Part model, mm, in its own coordinate system. Coordinates: 2 decimals unless noted, no trailing zeros. Order: outer loops, then holes, each group sorted by start corner. A loop starts at its lowest first (then second) coordinate and runs counter-clockwise, first axis right, second up. Notation, with made-up numbers: M 48,11 L 60,11 A20 ccw 60,20 Z; hole C 40.5,64 d1. An arc over 180 degrees is marked long. Answer in a Markdown table with one row per item. Add a question column.
Autodesk Inventor part; units mm, degrees
ref_plane "Work Plane2" through (18, 0, 0) normal (1, 0, 0) x (0, 1, 0)
ref_plane "XZ Plane" through (0, 0, 0) normal (0, 1, 0) x (-1, 0, 0)
ref_plane "XY Plane" through (0, 0, 0) normal (0, 0, 1) x (1, 0, 0)
sketch "Sketch3" plane through (0, 0, 0) normal (1, 0, 0) x (0, 1, 0)
  arc A0 (0, -20) -> (0, 20) centre (0, 0) ccw
  line L0 (0, 20) -> (0, -20)
  line L1 (0, -28) -> (0, 28)
  dimension "d15" = 20
revolve "Revolution4" add sketch "Sketch3" angle 360 about axis through (0, 0, -10) along (0, 0, 1)
ref_plane "Work Plane2" through (18, 0, 0) normal (1, 0, 0) x (0, 1, 0)
sketch "Sketch4" plane through (18, 0, 0) normal (1, 0, 0) x (0, 1, 0)
  circle A0 centre (0, 0) radius 8.4531
  circle A1 centre (0, 0) radius 4.5
  dimension "d20" = 9
extrude "Extrusion4" cut sketch "Sketch4" along normal through all contours A0 | A1
hole "Hole1" at (18, 0, 0) direction (-1, 0, 0) diameter 9 depth 10 tip angle 118
thread "Thread1"
properties part number "Knob" material "Iron, Cast"
(1) Slice it at D-D (x = -5.5). List the corners of the cut face in (y, z), and give its area (3 significant figures).
(2) Slice it at A-A (y = -13.5). List the corners of the cut face in (x, z), and give its area (3 significant figures).
(3) Drop flat-ended pins along their axis: P1, Ø10, axis at x = 2, z = 1, coming from the +Y side; P2, Ø3, axis at y = -8.5, z = 1.5, coming from the +X side; P3, Ø8, axis at x = 15, z = -7, coming from the -Y side; P4, Ø1.5, axis at y = 0, z = 11, coming from the -X side. Give the stop position or say it passes through.
(4) Slice it at C-C (x = 13). List the corners of the cut face in (y, z), and give its area (3 significant figures).
(5) Wall check: line 1 (Z direction, x = 10, y = 0); line 2 (Z direction, x = 13.25, y = 0); line 3 (Y direction, x = -2.5, z = 15). Give the ranges that are in metal, low to high.
(6) Slice it at B-B (z = 6.5). List the corners of the cut face in (x, y).
Computed:
| question | item | result |
|---|---|---|
| 1 | outline | C 0,0 d38.46 |
| 1 | area | 1,160 mm^2 |
| 2 | outline | C 0,0 d29.51 |
| 2 | area | 684 mm^2 |
| 3 | P1 | stops at y = 20 |
| 3 | P2 | stops at x = 18.13 |
| 3 | P3 | stops at y = -15.57 |
| 3 | P4 | stops at x = -17.17 |
| 4 | outline | C 0,0 d30.4; hole C 0,0 d9 |
| 4 | area | 662 mm^2 |
| 5 | line 1 | z = -17.32 to -4.5, 4.5 to 17.32 |
| 5 | line 2 | z = -14.98 to -4.5, 4.5 to 14.98 |
| 5 | line 3 | y = -12.99 to 12.99 |
| 6 | outline | M 18,-5.4 L 18,5.4 L 18.13,5.4 A18.91 ccw long 18.13,-5.4 Z |
